Build history of the part. All positions in model axes, mm. A direction names the side the tool comes from. Coordinates: 2 decimals unless noted, no trailing zeros. Order: outer loops, then holes, each group sorted by start corner. A loop starts at its lowest first (then second) coordinate and runs counter-clockwise, first axis right, second up. Notation, with made-up numbers: (-21, 89.25) - (24, 89.25) arc R30 cw to (24, 120.25) - close; hole circle Ø9 at (-9.75, 60.5). An arc over 180 degrees is marked (long way). Answer as CSV lines item,"result". Start each with the question number.
from build123d import *

# Parameters (mm, degrees)
EXTRUDE_3_DEPTH     = 240
EXTRUDE_5_DEPTH     = 100
SKETCH_9_W          = 30
SKETCH_9_H          = 170
CUT_EXTRUDE_1_DEPTH = 60
EXTRUDE_6_DEPTH     = 20


with BuildPart() as part:
    # 草图1 → 凸台-拉伸3 (new body)
    with BuildSketch(Plane.XY):
        Polygon((24.986954743, -11.866003736), (-5.013045257, -11.866003736), (-5.013045257, -1.866003736), (-0.013045257, -1.866003736), (-0.013045257, 8.133996264), (19.986954743, 8.133996264), (19.986954743, -1.866003736), (24.986954743, -1.866003736), align=None)
    extrude(amount=EXTRUDE_3_DEPTH)

    # 草图4 → 凸台-拉伸5 (add)
    with BuildSketch(Plane(origin=(0, 0, 0), x_dir=(-1, 0, 0), z_dir=(0, 0, -1))):
        Polygon((-19.986954743, 8.133996264), (0.013045257, 8.133996264), (0.013045257, -1.866003736), (5.013045257, -1.866003736), (5.013045257, -11.866003736), (-24.986954743, -11.866003736), (-24.986954743, -1.866003736), (-19.986954743, -1.866003736), align=None)
    extrude(amount=EXTRUDE_5_DEPTH)

    # 草图9 → 切除-拉伸1 (cut)
    with BuildSketch(Plane.XZ.offset(11.866003736)):
        with Locations((9.986954743, -15)):
            Rectangle(SKETCH_9_W, SKETCH_9_H)
    extrude(amount=-CUT_EXTRUDE_1_DEPTH, mode=Mode.SUBTRACT)

    # 草图11 → 凸台-拉伸6 (add)
    with BuildSketch(Plane(origin=(19.986954743, 0, 0), x_dir=(0, 0, -1), z_dir=(1, 0, 0))):
        with BuildLine():
            ThreePointArc((-145, 18.133996264), (-155, 28.133996264), (-165, 18.133996264))
            Line((-165, 18.133996264), (-158, 18.133996264))
            ThreePointArc((-158, 18.133996264), (-155, 21.133996264), (-152, 18.133996264))
            Line((-152, 18.133996264), (-145, 18.133996264))
        make_face()
        with BuildLine():
            Line((-158, 18.133996264), (-165, 18.133996264))
            ThreePointArc((-165, 18.133996264), (-162.071067812, 11.062928453), (-155, 8.133996264))
            ThreePointArc((-155, 8.133996264), (-147.928932188, 11.062928453), (-145, 18.133996264))
            Line((-145, 18.133996264), (-152, 18.133996264))
            ThreePointArc((-152, 18.133996264), (-155, 15.133996264), (-158, 18.133996264))
        make_face()
        with BuildLine():
            ThreePointArc((-145, 18.133996264), (-147.928932188, 11.062928453), (-155, 8.133996264))
            Line((-155, 8.133996264), (-145, 8.133996264))
            Line((-145, 8.133996264), (-145, 18.133996264))
        make_face()
        with BuildLine():
            Line((-165, 18.133996264), (-165, 8.133996264))
            Line((-165, 8.133996264), (-155, 8.133996264))
            ThreePointArc((-155, 8.133996264), (-162.071067812, 11.062928453), (-165, 18.133996264))
        make_face()
    extrude(amount=-EXTRUDE_6_DEPTH)


solid = part.part
(1) Band-saw the part on D-D on x = 21.5. List the corners of the cut face in (y, z), plus the area to 3 significant figures.
(2) Drop flat-ended pins along their axis: pin 1 Ø10 at (x, z) = (7, 114.5) entering from +Y; pin 2 Ø5 at (x, y) = (9.5, 13) entering from -Z; pin 3 Ø2 at (y, z) = (5.5, 152) entering from -X. Give the stop position or say it passes through.
(3) Probe L1, parallel to Y at x = 9.5, z = 155; L2, parallel to X at y = 7.5, z = 136; L3, parallel to Y at x = -0.75, z = 100. List the from-to ranges inside material, lowest first. Write a range as [from, to].
(4) Band-saw the part on B-B on x = 12.25. List the corners of the cut face in (y, z).
(5) Pull direction Y, two halves, no side cores. Call faces 1 (the flat face through (-2, -1.866, 156)), 2 (the cylindrical face through (10.13, 19.04, 157.86)), 3 (the flat face through (10, 13, 145)): +Y half, -Y half, draft (parallel to the pull), parting line (faces both ways), or undercut.
(6) Band-saw the part on A-A on z = 155. List the corners of the cut face in (x, y).
(7) Which spindle directions (+Z, -Z, +X, -X, +Y, -Y) get a long thin tool onto all of the face, cutting with end or side? Do faces 4 (the flat face through (23, -1.866, 156)), 5 (the flat face through (10, 8.134, 108)), 6 (the flat face through (10, 13, 165)), 7 (the flat face through (10, -2, 70)), 8 (the flat face through (-0.013, 7, 156)). Say none if no direction does.
(8) Band-saw the part on C-C on z = 174. List the corners of the cut face in (x, y).
Filled in:
1,outline,"(-11.87, 70) - (-1.87, 70) - (-1.87, 240) - (-11.87, 240) - close"
1,area,"1,700 mm^2"
2,pin 1,"stops at y = 8.13"
2,pin 2,"stops at z = 145"
2,pin 3,"stops at x = -0.01"
3,L1,"y = [-11.87, 15.13], [21.13, 28.13]"
3,L2,"x = [-0.01, 19.99]"
3,L3,"y = [-11.87, -1.87]"
4,outline,"(-11.87, 70) - (8.13, 70) - (8.13, 145) - (18.13, 145) arc R10 ccw to (18.13, 165) - (8.13, 165) - (8.13, 240) - (-11.87, 240) - close; hole circle Ø6 at (18.13, 155)"
5,face 1,"+Y half"
5,face 2,"undercut"
5,face 3,"draft"
6,outline,"(-5.01, -11.87) - (24.99, -11.87) - (24.99, -1.87) - (19.99, -1.87) - (19.99, 15.13) - (-0.01, 15.13) - (-0.01, -1.87) - (-5.01, -1.87) - close; (-0.01, 21.13) - (19.99, 21.13) - (19.99, 28.13) - (-0.01, 28.13) - close"
7,face 4,"+Z, -Z, +X, +Y"
7,face 5,"-Z, +X, -X, +Y"
7,face 6,"+Z, +X, -X, +Y"
7,face 7,"-Z, +X, -X, +Y, -Y"
7,face 8,"+Z, -Z, -X, +Y"
8,outline,"(-5.01, -11.87) - (24.99, -11.87) - (24.99, -1.87) - (19.99, -1.87) - (19.99, 8.13) - (-0.01, 8.13) - (-0.01, -1.87) - (-5.01, -1.87) - close"
